Answer from the drawing. Dimensions are ordinates in mm from the lowest x, y and z of the part. Round coordinates to 2 decimals unless told otherwise and drop trailing zeros. Order: outer loops, then holes, each group sorted by start corner. A loop starts at its lowest first (then second) coordinate and runs counter-clockwise, first axis right, second up. Notation, with made-up numbers: M -6.75,86.5 L 7.25,86.5 A5 cw 7.25,95.5 Z; hole C 6.25,68 d2. An arc over 180 degrees is marked long. Answer as a JSON object with one key per item and string values. Group by question number.
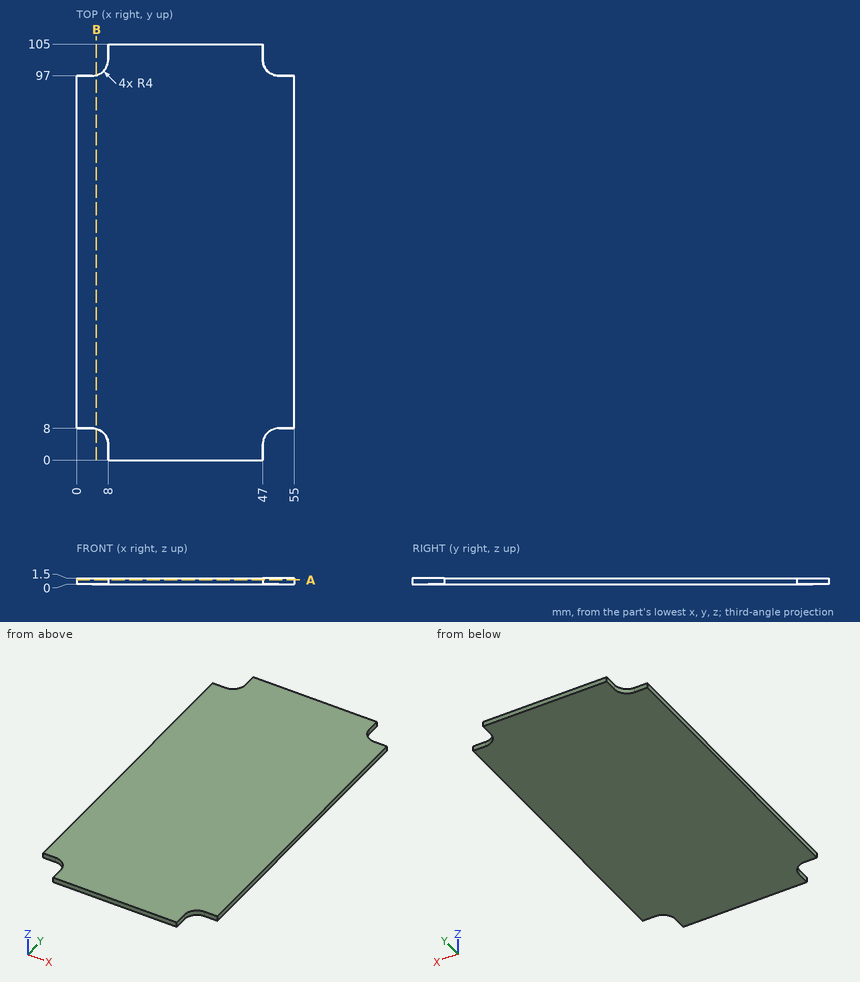
Item 1: Find section B-B (x = 5). Give the vertices of the cut face in (y, z).
Item 2: Consider L1, parallel to Y at x = 2, z = 0.7; L2, parallel to Y at x = 49.5, z = 1.25. Determine where each line is inside the solid, lowest interval first.
Item 3: Find section A-A (z = 1.05). Give the vertices of the cut face in (x, y).
Item 4: Each of these flat-tipped pins is pushed along its axis until it touches: pin 1 (0.8 mm diameter, centred on x = 52, z = 0.5, fed in from +Y); pin 2 (1 mm diameter, centred on x = 10.5, y = 56.5, fed in from -Z). Where does it stop, or does it pass through?
Responses:
{
 "1": {"outline": "M 7.87,0 L 97.13,0 L 97.13,1.5 L 7.87,1.5 Z"},
 "2": {"L1": "y = 8 to 97", "L2": "y = 7.71 to 97.29"},
 "3": {"outline": "M 0,8 L 4,8 A4 cw 8,4 L 8,0 L 47,0 L 47,4 A4 cw 51,8 L 55,8 L 55,97 L 51,97 A4 cw 47,101 L 47,105 L 8,105 L 8,101 A4 cw 4,97 L 0,97 Z"},
 "4": {"pin 1": "stops at y = 97", "pin 2": "stops at z = 0"}
}
